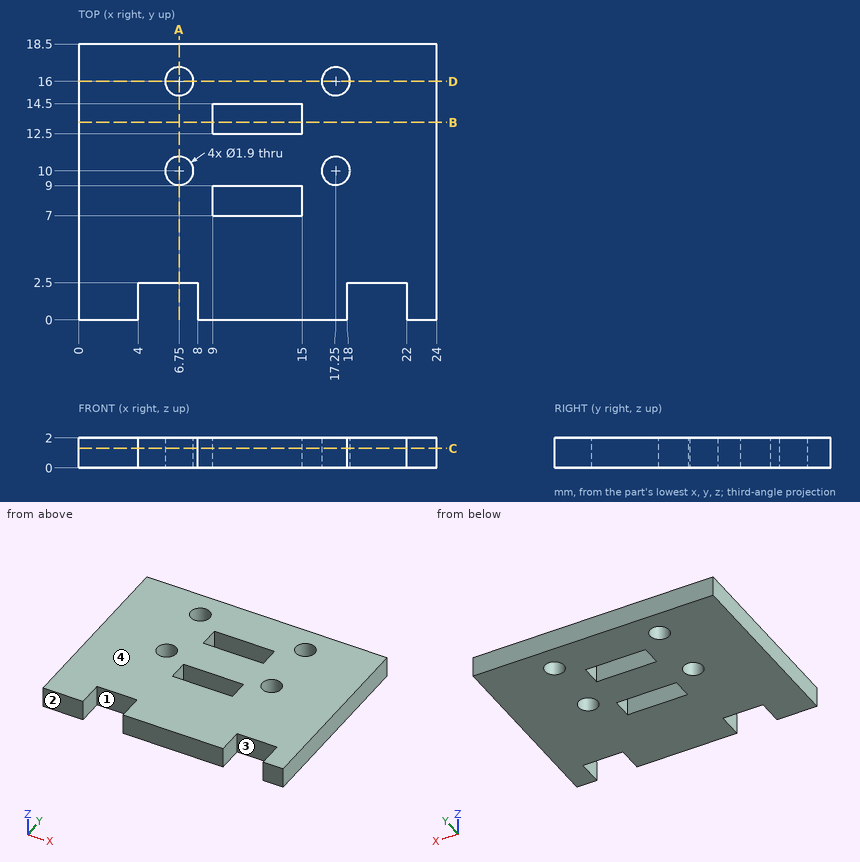
Here's the drawing with two shaded views (mm, measured from the low corner). I have some questions. A direction names the side the tool comes from. Coordinates: 2 decimals unless noted, no trailing zeros. Order: outer loops, then holes, each group sorted by start corner. A loop starts at its lowest first (then second) coordinate and runs counter-clockwise, first axis right, second up.
Q1. Which directions (+Z, -Z, +X, -X, +Y, -Y) give clear straight access to the entire face, cutting with the end or side of a thin tool? Please do the marked faces 3 and 4.
Q2. Suppose I cut it at B-B on y = 13.25. Please give me the cut outline in (x, z), and give its area (3 significant figures).
Q3. Suppose I cut it at A-A on x = 6.75. Please give me the cut outline in (y, z), and give its area (3 significant figures).
Q4. Will this pin go through, and if not, where does the flat tip stop? pin 1 (0.6 mm diameter, centred on x = 5.5, z = 1.5, fed in from -Y).
Q5. Suppose I cut it at D-D on y = 16. Please give me the cut outline in (x, z).
Q6. Please list where these lines run through material, in increasing order: L1, parallel to Y at x = 12, z = 1.35; L2, parallel to Y at x = 17.25, z = 0.8; L3, parallel to X at y = 2.25, z = 0.45.
Q7. Suppose I cut it at C-C on z = 1.3. Please give me the cut outline in (x, y).
Q8. Thinking about a two-plate mould opening in X: for the marked faces 1 and 2, which applies, released by +X, released by -X, zero draft, split by the parting line, or undercut?
Answer:
1. face 3: +Z, -Z, -Y
1. face 4: +Z, +X, -X, +Y, -Y
2. outline: (0, 0) - (9, 0) - (9, 2) - (0, 2) - close; (15, 0) - (24, 0) - (24, 2) - (15, 2) - close
2. area: 36.0 mm2
3. outline: (2.5, 0) - (9.05, 0) - (9.05, 2) - (2.5, 2) - close; (10.95, 0) - (15.05, 0) - (15.05, 2) - (10.95, 2) - close; (16.95, 0) - (18.5, 0) - (18.5, 2) - (16.95, 2) - close
3. area: 24.4 mm2
4. pin 1: stops at y = 2.5
5. outline: (0, 0) - (5.8, 0) - (5.8, 2) - (0, 2) - close; (7.7, 0) - (16.3, 0) - (16.3, 2) - (7.7, 2) - close; (18.2, 0) - (24, 0) - (24, 2) - (18.2, 2) - close
6. L1: y = 0 to 7, 9 to 12.5, 14.5 to 18.5
6. L2: y = 0 to 9.05, 10.95 to 15.05, 16.95 to 18.5
6. L3: x = 0 to 4, 8 to 18, 22 to 24
7. outline: (0, 0) - (4, 0) - (4, 2.5) - (8, 2.5) - (8, 0) - (18, 0) - (18, 2.5) - (22, 2.5) - (22, 0) - (24, 0) - (24, 18.5) - (0, 18.5) - close; hole circle Ø1.9 at (6.75, 10); hole circle Ø1.9 at (6.75, 16); hole (9, 7) - (15, 7) - (15, 9) - (9, 9) - close; hole (9, 12.5) - (15, 12.5) - (15, 14.5) - (9, 14.5) - close; hole circle Ø1.9 at (17.25, 10); hole circle Ø1.9 at (17.25, 16)
8. face 1: undercut
8. face 2: zero draft
